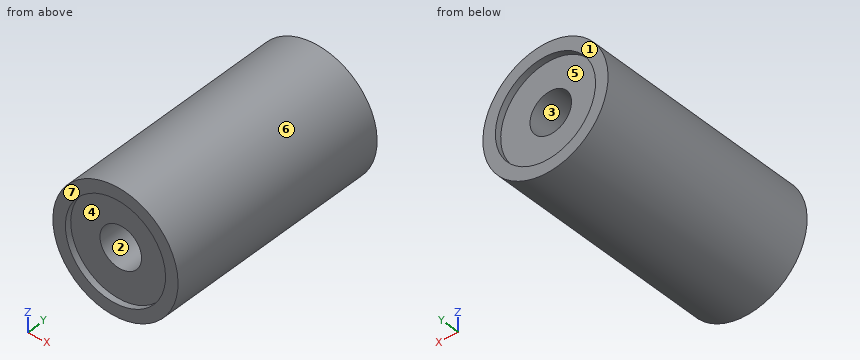
from build123d import *

# Parameters (mm, degrees)
BOSS_EXTRUDE1_DEPTH      = 23.8125
BOSS_EXTRUDE1_DEPTH_BACK = 23.8125
SKETCH1_R                = 12.7
SKETCH2_R                = 10.16
CUT_EXTRUDE1_DEPTH       = 1.27


with BuildPart() as part:
    # Sketch1 → Boss-Extrude1 (new, two sides: drawn at the far end of the back side and taken through both)
    with BuildSketch(Plane(origin=(0, 0, 0), x_dir=(1, 0, 0), z_dir=(0, 1, 0)).offset(-BOSS_EXTRUDE1_DEPTH_BACK)):
        with Locations(Location((0, 0, 0), (0, 0, 270))):
            Circle(SKETCH1_R)
    extrude(amount=BOSS_EXTRUDE1_DEPTH + BOSS_EXTRUDE1_DEPTH_BACK)

    # Sketch2 → Cut-Extrude1 (cut)
    with BuildSketch(Plane(origin=(0, 23.8125, 0), x_dir=(1, 0, 0), z_dir=(0, 1, 0))):
        with Locations(Location((0, 0, 0), (0, 0, 270))):
            Circle(SKETCH2_R)
    cut_extrude1 = extrude(amount=-CUT_EXTRUDE1_DEPTH, mode=Mode.SUBTRACT)

    # Sketch5 → 3_8-24 Tapped Hole1 (revolve, cut)
    with BuildSketch(Plane(origin=(0, 22.5425, 0), x_dir=(0, 0, 1), z_dir=(1, 0, 0))):
        Polygon((0, 0), (0, 18.535468714), (4.2164, 16.002), (4.2164, 0), align=None)
    f_3_8_24_tapped_hole1 = revolve(axis=Axis((0, 28.8925, 0), (0, -1, 0)), mode=Mode.SUBTRACT)

    # Mirror1: Cut-Extrude1, 3_8-24 Tapped Hole1 across plane
    add(cut_extrude1.mirror(Plane.ZX), mode=Mode.SUBTRACT)
    add(f_3_8_24_tapped_hole1.mirror(Plane.ZX), mode=Mode.SUBTRACT)


solid = part.part
Could you check a few things on this model? Use its own coordinates, in mm. Face numbers are marked on the shaded views. A direction names the side the tool comes from. Give positions to 0.01 mm unless a question says otherwise; leave off trailing zeros. Order: outer loops, then holes, each group sorted by start corner. A loop starts at its lowest first (then second) coordinate and runs counter-clockwise, first axis right, second up. Notation, with made-up numbers: (17.5, -15) - (44.5, -15) arc R13 cw to (44.5, 0) - close; hole circle Ø4 at (-15, 19). An arc over 180 degrees is marked (long way). Return JSON: item names as keys, results as strings. Group by question number.
Q1. Suppose I cut it at C-C, the plane x = 11. Please give me the cut outline in (y, z), and give its area (3 significant figures).
Q2. Suppose I cut it at A-A, the plane z = -9.5. Please give me the cut outline in (x, y), and give its area (3 significant figures).
Q3. Which directions (+Z, -Z, +X, -X, +Y, -Y) give clear straight access to the entire face, cutting with the end or side of a thin tool? Please do the marked faces 1, 2 and 3.
Q4. Thinking about a two-plate mould opening in X: for the marked faces 4, 5, 6 and 7, which applies, pulls with the +X half, pulls with the -X half, needs draft (parallel to the pull), parting line crosses it, or undercut?
Q5. Suppose I cut it at B-B, the plane y = -11. Please give me the cut outline in (x, z).
Q6. Suppose I cut it at D-D, the plane z = 7. Please give me the cut outline in (x, y), and give its area (3 significant figures).
Q7. Please list where these lines run through material, in increasing order: line 1 along X through (y, z) = (-23.35, 0); line 2 along X through (y, z) = (-18, 0); line 3 along Z through (x, y) = (0.5, 20). Write a range as [from, to].
Q8. Will these pins go through, and if not, where does the flat tip stop? pin 1 Ø11 at (x, z) = (0, 0) entering from -Y; pin 2 Ø10 at (y, z) = (3, -6.5) entering from +X; pin 3 Ø5 at (x, y) = (3, -11) entering from -Z.
Resolved:
{
 "1": {"outline": "(-23.81, -6.35) - (23.81, -6.35) - (23.81, 6.35) - (-23.81, 6.35) - close", "area": "605 mm2"},
 "2": {"outline": "(-8.43, -23.81) - (-3.6, -23.81) - (-3.6, -22.54) - (3.6, -22.54) - (3.6, -23.81) - (8.43, -23.81) - (8.43, 23.81) - (3.6, 23.81) - (3.6, 22.54) - (-3.6, 22.54) - (-3.6, 23.81) - (-8.43, 23.81) - close", "area": "785 mm2"},
 "3": {"face 1": "+Z, -Z, +X, -X, +Y", "face 2": "-Y", "face 3": "+Y"},
 "4": {"face 4": "undercut", "face 5": "undercut", "face 6": "parting line crosses it", "face 7": "needs draft"},
 "5": {"outline": "circle Ø25.4 at (0, 0); hole circle Ø8.43 at (0, 0)"},
 "6": {"outline": "(-10.6, -23.81) - (-7.36, -23.81) - (-7.36, -22.54) - (7.36, -22.54) - (7.36, -23.81) - (10.6, -23.81) - (10.6, 23.81) - (7.36, 23.81) - (7.36, 22.54) - (-7.36, 22.54) - (-7.36, 23.81) - (-10.6, 23.81) - close", "area": "972 mm2"},
 "7": {"line 1": "x = [-12.7, -10.16], [10.16, 12.7]", "line 2": "x = [-12.7, -4.22], [4.22, 12.7]", "line 3": "z = [-12.69, -4.19], [4.19, 12.69]"},
 "8": {"pin 1": "stops at y = -22.54", "pin 2": "stops at x = 12.61", "pin 3": "stops at z = -12.69"}
}
